Source: CAD feature listing. Evaluate the final solid. Frame: model axes, mm. Give positions to 0.01 mm unless a question says otherwise; leave off trailing zeros. Order: outer loops, then holes, each group sorted by start corner. A loop starts at its lowest first (then second) coordinate and runs counter-clockwise, first axis right, second up. Notation, with made-up numbers: M 35.5,30 L 56.5,30 A18 cw 56.5,41 Z; hole C -32.75,59 d8. An arc over 180 degrees is marked long. Return JSON: item names as keys, results as strings.
Autodesk Inventor part; units mm, degrees
ref_plane "Work Plane1" through (-75, 0, -51) normal (0, 0, 1) x (1, 0, 0)
ref_plane "Work Plane2" through (-40, 0, 13) normal (1, 0, 0) x (0, 0, -1)
ref_plane "YZ Plane" through (0, 0, 0) normal (1, 0, 0) x (0, 1, 0)
sketch "Sketch1" plane through (0, 0, 0) normal (0, 1, 0) x (-1, 0, 0)
  line L0 (-15, 33) -> (95, 33)
  line L1 (95, 33) -> (95, -135)
  line L2 (95, -135) -> (-15, -135)
  line L3 (-15, -135) -> (-15, 33)
  line L4 (95, 33) -> (95, 15)
  line L5 (-15, 33) -> (-15, 13)
  line L6 (95, -135) -> (95, -115)
  line L7 (-15, -135) -> (-15, -115)
  line L8 (40, -135) -> (40, -130)
  line L9 (31, -130) -> (49, -130)
  line L10 (49, -130) -> (49, -106)
  line L11 (49, -106) -> (31, -106)
  line L12 (31, -106) -> (31, -130)
  line L13 (40, 33) -> (40, 28)
  line L14 (31, 28) -> (49, 28)
  line L15 (49, 28) -> (49, 4)
  line L16 (49, 4) -> (31, 4)
  line L17 (31, 4) -> (31, 28)
  point P0 (0, 0)
  point P1 (47.5, 33)
  point P2 (12.5, 33)
  point P3 (67.5, -135)
  point P4 (32.5, -135)
  dimension "d4" = 110
  dimension "d5" = 168
  dimension "d22" = 5
  dimension "d23" = 18
  dimension "d24" = 24
  dimension "d25" = 5
  dimension "d26" = 18
  dimension "d27" = 24
extrude "Extrusion2" add sketch "Sketch1" along normal blind 3 contours L9 L12 L11 L10 | L14 L15 L16 L17 | L0 L1 L2 L3
fillet "Fillet1" radius 20 4 edges at (15, 1.5, 33) (-95, 1.5, 33) (15, 1.5, -135) (-95, 1.5, -135)
ref_plane "Work Plane1" through (-75, 0, -51) normal (0, 0, 1) x (1, 0, 0)
ref_plane "Work Plane2" through (-40, 0, 13) normal (1, 0, 0) x (0, 0, -1)
sketch "Sketch2" plane through (0, 3, 0) normal (0, 1, 0) x (1, 0, 0)
  arc A0 (-95, -13) -> (-75, -33) centre (-75, -13) ccw
  line L0 (-95, -33) -> (-95, -13)
  line L1 (-75, -33) -> (-5, -33)
  line L2 (-95, -33) -> (-75, -33)
  line L3 (-75, -33) -> (-75, -13)
  line L4 (-75, -13) -> (-95, -13)
  arc A1 (-5, -33) -> (15, -13) centre (-5, -13) ccw
  line L5 (15, -33) -> (-5, -33)
  line L6 (15, -33) -> (15, -13)
  line L7 (-5, -33) -> (-5, -13)
  line L8 (-5, -13) -> (15, -13)
  arc A2 (15, 115) -> (-5, 135) centre (-5, 115) ccw
  line L9 (15, 135) -> (15, 115)
  line L10 (15, 135) -> (-5, 135)
  line L11 (-5, 135) -> (-5, 115)
  line L12 (-5, 115) -> (15, 115)
  arc A3 (-75, 135) -> (-95, 115) centre (-75, 115) ccw
  line L13 (-95, 135) -> (-95, 115)
  line L14 (-95, 135) -> (-75, 135)
  line L15 (-95, 115) -> (-95, -13)
  line L16 (-95, 115) -> (-75, 115)
  line L17 (-75, 115) -> (-75, 135)
  point P0 (0, 0)
hole "Hole2" at (-75, 3, 13) at (-75, 3, -115) at (-5, 3, -115) at (-5, 3, 13) direction (0, -1, 0) diameter 4.3 end through all
properties part number "BedHousingFrame"
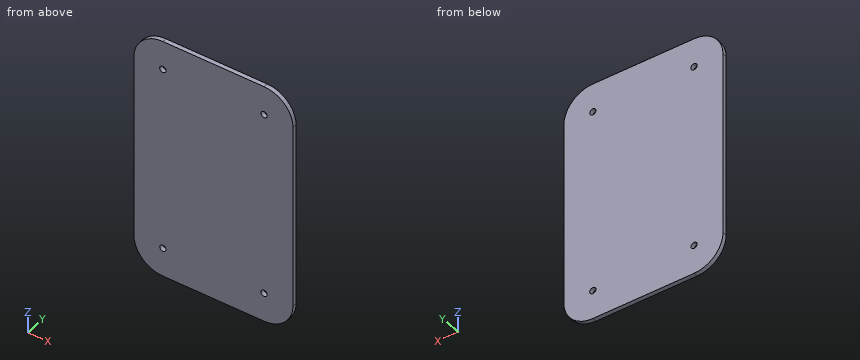
1. Section query B-B (x = 4.5). Return loops of the section in (y, z), then the cut area to 3 significant figures.
Evaluation:
{"outline": "M 0,-132.6 L 3,-132.6 L 3,30.6 L 0,30.6 Z", "area": "490 mm^2"}
2. Section query A-A (y = 2.5). Return loops of the section in (x, z).
Evaluation:
{"outline": "M -95,-115 A20 ccw -75,-135 L -5,-135 A20 ccw 15,-115 L 15,13 A20 ccw -5,33 L -75,33 A20 ccw -95,13 Z; hole C -75,-115 d4.3; hole C -75,13 d4.3; hole C -5,-115 d4.3; hole C -5,13 d4.3"}
3. Ray query, probe 1 along X at (y, z) = (1.4, 13); probe 2 along Z at (x, y) = (-5, 1.2); probe 3 along X at (y, z) = (1.15, -114). Return the intervals inside material, ascending.
Evaluation:
{"probe 1": "x = -95 to -77.15, -72.85 to -7.15, -2.85 to 15", "probe 2": "z = -135 to -117.15, -112.85 to 10.85, 15.15 to 33", "probe 3": "x = -95 to -76.9, -73.1 to -6.9, -3.1 to 15"}
